from build123d import *

# Parameters (mm, degrees)
F0_R     = 13.75
F1_DEPTH = 47
F2_R     = 13.75
F3_DEPTH = 9.5
F4_R     = 8
F5_DEPTH = 56.501
F7_D     = 5.5


with BuildPart() as f1:
    # F0 (on Front) → F1 (new body)
    with BuildSketch(Plane.XZ):
        Circle(F0_R)
    extrude(amount=F1_DEPTH)

    # F2 (on face) → F3 (join)
    with BuildSketch(Plane.XZ.offset(47)):
        with BuildLine():
            Line((13.0264154701, 20.75), (-13.0264154701, 20.75))
            ThreePointArc((-13.0264154701, 20.75), (-24.5, 0), (-13.0264154701, -20.75))
            Line((-13.0264154701, -20.75), (13.0264154701, -20.75))
            ThreePointArc((13.0264154701, -20.75), (24.5, 0), (13.0264154701, 20.75))
        make_face()
        Circle(F2_R, mode=Mode.SUBTRACT)
        Circle(F2_R)
    extrude(amount=F3_DEPTH)

    # F4 (on face) → F5 (cut, through all)
    with BuildSketch(Plane.XZ.offset(56.5)):
        Circle(F4_R)
    extrude(amount=-F5_DEPTH, mode=Mode.SUBTRACT)

    # F7 (through all)
    with Locations(Plane.XZ.offset(56.5)):
        with Locations((-16.4544826719, 9.5), (-16.4544826719, -9.5), (16.4544826719, 9.5), (16.4544826719, -9.5)):
            Hole(F7_D / 2)


solid = f1.part
Check sheet for the modelled part. Datum: model origin and axes. Units: mm. A direction names the side the tool comes from. Coordinates: 2 decimals unless noted, no trailing zeros. Write each loop counter-clockwise with the first axis right and the second up, starting at its lowest first coordinate (ties: lowest second). Pieces come first, ordered by that corner, then holes.
Item 1: Mould release check, pull along Z, two halves, no side actions. Record for faces 3 (the face through (-13.707, -51.683, -9.379)), 4 (the face through (0, -52, -20.75)), 5 (the face through (0, -52, 20.75)), 6 (the face through (18.64, -51.68, -11.17)): released by +Z, released by -Z, zero draft, split by the parting line, or undercut.
Numbers:
face 3: undercut
face 4: released by -Z
face 5: released by +Z
face 6: undercut
Item 2: Depth check by flat-ended pin: pin 1 Ø2 at (y, z) = (-26, 4.5) entering from -X; pin 2 Ø1 at (x, y) = (7, -29) entering from +Z; pin 3 Ø1.5 at (y, z) = (-50.5, -7) entering from -X. Enter the tip coordinate at first touch or a pass-through.
Numbers:
pin 1: stops at x = -13.3
pin 2: stops at z = 12.12
pin 3: stops at x = -23.69
Item 3: Cross-section at C-C on z = 9.5. Record the boundary of the cut face in (x, y), then the cut area to 3 significant figures.
Numbers:
outline: (-22.58, -56.5) - (-19.2, -56.5) - (-19.2, -47) - (-22.58, -47) - close; (-13.7, -56.5) - (13.7, -56.5) - (13.7, -47) - (9.94, -47) - (9.94, 0) - (-9.94, 0) - (-9.94, -47) - (-13.7, -47) - close; (19.2, -56.5) - (22.58, -56.5) - (22.58, -47) - (19.2, -47) - close
area: 1,260 mm2
Item 4: Scan lines: probe 1 along X at (y, z) = (-50, -11.5); probe 2 along X at (y, z) = (-51, -9); probe 3 along Z at (x, y) = (0, -22.5). Record each from-to range of solid material in increasing order.
Numbers:
probe 1: x = -21.63 to -18.34, -14.57 to 14.57, 18.34 to 21.63
probe 2: x = -22.79 to -19.16, -13.75 to 13.75, 19.16 to 22.79
probe 3: z = -13.75 to -8, 8 to 13.75
Item 5: Access from +Z, -Z, +X, -X, +Y, -Y to the whole of each face (thin tool, end or side, straight path). Record for faces 1 (the face through (6, 0, -6)), 2 (the face through (-2.981, -23.171, -13.423)).
Numbers:
face 1: +Z, -Z, +X, -X, +Y
face 2: +Y
Item 6: Cross-section at A-A on z = 0. Record the boundary of the cut face in (x, y), then the cut area to 3 significant figures.
Numbers:
outline: (-24.5, -56.5) - (-8, -56.5) - (-8, 0) - (-13.75, 0) - (-13.75, -47) - (-24.5, -47) - close; (8, -56.5) - (24.5, -56.5) - (24.5, -47) - (13.75, -47) - (13.75, 0) - (8, 0) - close
area: 854 mm2
Item 7: Cross-section at B-B on x = -18.5. Record the boundary of the cut face in (y, z).
Numbers:
outline: (-56.5, -16.06) - (-47, -16.06) - (-47, -11.34) - (-56.5, -11.34) - close; (-56.5, -7.66) - (-47, -7.66) - (-47, 7.66) - (-56.5, 7.66) - close; (-56.5, 11.34) - (-47, 11.34) - (-47, 16.06) - (-56.5, 16.06) - close
Item 8: Cross-section at D-D on y = -11. Record the boundary of the cut face in (x, z).
Numbers:
outline: circle Ø27.5 at (0, 0); hole circle Ø16 at (0, 0)
